```python
from build123d import *

# Parameters (mm, degrees)
F1_DEPTH = 100
F2_W     = 80
F2_H     = 20
F3_DEPTH = 100
F4_W     = 80
F4_H     = 20
F5_DEPTH = 100
F6_R     = 5


with BuildPart() as f1:
    # F0 (on Front) → F1 (new body)
    with BuildSketch(Plane.XZ):
        Polygon((0, 50), (-50, -50), (-25.9177014232, -50), (-15.7341611385, -30), (-5.5506208539, -10), (25, -10), (25, -30), (25, -50), (50, -50), (50, -30), (50, -10), (50, 10), (50, 30), (50, 50), (25, 50), align=None)
        Polygon((14.8164597154, 30), (25, 30), (25, 10), (4.6329194307, 10), align=None, mode=Mode.SUBTRACT)
    extrude(amount=F1_DEPTH)

    # F2 (on face) → F3 (cut)
    with BuildSketch(Plane.YZ.offset(50)):
        with Locations((-60, -20)):
            Rectangle(F2_W, F2_H)
    extrude(amount=-F3_DEPTH, mode=Mode.SUBTRACT)

    # F4 (on face) → F5 (cut)
    with BuildSketch(Plane.YZ.offset(50)):
        with Locations((-40, 20)):
            Rectangle(F4_W, F4_H)
    extrude(amount=-F5_DEPTH, mode=Mode.SUBTRACT)

    # F6
    f6_edges = [f1.edges().sort_by_distance(p)[0] for p in [
        (50, -100, -40),
        (50, -100, 20),
        (50, -50, 50),
        (25, -100, 50),
        (0, -50, 50),
        (-15, -100, 20),
        (-45, -100, -40),
        (50, 0, -20),
        (50, 0, 40),
        (-35, 0, -20),
        (-5, 0, 40),
        (25, 0, 50),
    ]]
    fillet(f6_edges, radius=F6_R)


solid = f1.part
```
Here's how the part is built. I have some questions about the finished solid (model axes, mm). A direction names the side the tool comes from. Coordinates: 2 decimals unless noted, no trailing zeros. Loops run counter-clockwise (first coordinate to the right, second up) from the corner with the lowest first, then second, coordinate; pieces in that order, holes last. Notation, with made-up numbers: M 20.5,66 L 27.5,66 A16 cw 27.5,95 Z; hole C -10.5,-28 d8. An arc over 180 degrees is marked long. One line per item, written item: value.
1. On a 3-axis mill with a long thin cutter (end or side, diameter ignored), from which of +Z, -Z, +X, -X, +Y, -Y can I reach the whole of each face in a straight line? I mean faces 4 (the flat face through (25, -90, 20)), 5 (the flat face through (25, -38, -39)), 6 (the flat face through (-28, -61, -30)). Say none if no direction works.
Geometry says:
face 4: +Y, -Y
face 5: -Z, +Y, -Y
face 6: +X, -X, -Y
2. Imagine slicing it at C-C (y = -49). List the corners of the cut face in (x, z) for me.
Geometry says:
outline: M -50,-50 L -25.92,-50 L -15.73,-30 L -40,-30 Z; M -30,-10 L 50,-10 L 50,10 L -20,10 Z; M -10,30 L 50,30 L 50,45 A5 ccw 45,50 L 3.09,50 A5 ccw -1.38,47.24 Z; M 25,-50 L 50,-50 L 50,-30 L 25,-30 Z
3. Imagine slicing it at A-A (y = -10.5). List the corners of the cut face in (x, z) for me, and give its area (3 significant figures).
Geometry says:
outline: M -50,-50 L -25.92,-50 L -5.55,-10 L 25,-10 L 25,-50 L 50,-50 L 50,10 L -20,10 Z; M -10,30 L 50,30 L 50,45 A5 ccw 45,50 L 3.09,50 A5 ccw -1.38,47.24 Z
area: 4,560 mm2
4. Imagine slicing it at D-D (x = 41.5). List the corners of the cut face in (y, z) for me.
Geometry says:
outline: M -100,-50 L 0,-50 L 0,10 L -80,10 L -80,30 L 0,30 L 0,45 A5 ccw -5,50 L -95,50 A5 ccw -100,45 L -100,-10 L -20,-10 L -20,-30 L -100,-30 Z
5. Thinking about a two-plate mould opening in Z: for faces 1 (the flat face through (38, -20, -20)), 2 (the cylindrical face through (-43.24, -98.5, -39.68)), 3 (the cylindrical face through (49, -98, -40)), which applies, +Z half, -Z half, draft (parallel to the pull), parting line (faces both ways), or undercut?
Geometry says:
face 1: undercut
face 2: +Z half
face 3: draft
6. Imagine slicing it at B-B (x = 20.5). List the corners of the cut face in (y, z) for me.
Geometry says:
outline: M -100,-10 L 0,-10 L 0,10 L -100,10 Z; M -100,30 L 0,30 L 0,45 A5 ccw -5,50 L -95,50 A5 ccw -100,45 Z
7. Please list where these lines run through material, in increasing order: probe 1 along Z at (x, y) = (35, -37.5); probe 2 along Z at (x, y) = (18, -71.5); probe 3 along Z at (x, y) = (-11, -40).
Geometry says:
probe 1: z = -50 to -30, -10 to 10, 30 to 50
probe 2: z = -10 to 10, 30 to 50
probe 3: z = -10 to 10
8. Will these pins go through, and if not, where does the flat tip stop? pin 1 Ø5 at (x, y) = (0, -39) entering from -Z; pin 2 Ø2 at (x, z) = (-23.5, 2) entering from -Y; pin 3 Ø6 at (x, z) = (-22.5, -21.5) entering from -Y.
Geometry says:
pin 1: stops at z = -10
pin 2: stops at y = -98.52
pin 3: stops at y = -20
